For this review, take the finished solid that the model builds, in its own axes (mm). Coordinates: 2 decimals unless noted, no trailing zeros. Loops run counter-clockwise (first coordinate to the right, second up) from the corner with the lowest first, then second, coordinate; pieces in that order, holes last.
1. Take a section at B-B, the plane z = -371. State the section outline as (x, y) points, then the cut area to 3 significant figures.
2. Clearance check with flat-ended pins moving along their axes: P1, Ø12.5, axis at y = 743.5, z = -1133.5, coming from the +X side; P2, Ø23, axis at x = 364, y = 55, coming from the -Z side; P3, Ø12.5, axis at y = 755, z = -111.5, coming from the -X side. State where each tip first meets the part, or that it passes through.
3. To check wall thickness, follow probe 1 along Y at (x, z) = (1123, -1114); probe 2 along Y at (x, z) = (302, -77); probe 3 along Z at (x, y) = (80, 551). State the ranges of each line that lie inside material, in increasing order.
4. Take a section at C-C, the plane y = 277.5. State the section outline as (x, z) points, then the cut area to 3 significant figures.
5. Take a section at A-A, the plane x = 207.5. State the section outline as (y, z) points.
```python
from build123d import *

# Parameters (mm, degrees)
SKETCH1_W               = 1219.2
SKETCH1_H               = 1219.2
BOSS_EXTRUDE1_DEPTH     = 25.4
SKETCH2_W               = 76.2
SKETCH2_H               = 76.2
BOSS_EXTRUDE2_DEPTH     = 711.2
BOSS_EXTRUDE3_REACH     = 1812.541
SKETCH3_W               = 76.2
SKETCH3_H               = 76.2
BOSS_EXTRUDE4_REACH     = 1812.541
SKETCH4_W               = 76.2
SKETCH4_H               = 76.2
SKETCH5_W               = 127
SKETCH5_H               = 127
BOSS_EXTRUDE5_DEPTH     = 25.4
F_1_2_13_TAPPED_HOLE1_D = 10.71626


with BuildPart() as part:
    # Sketch1 → Boss-Extrude1 (new body)
    with BuildSketch(Plane(origin=(0, 0, 0), x_dir=(1, 0, 0), z_dir=(0, 1, 0))):
        with Locations((609.6, 609.6)):
            Rectangle(SKETCH1_W, SKETCH1_H)
    extrude(amount=BOSS_EXTRUDE1_DEPTH)

    # Sketch2 → Boss-Extrude2 (add)
    with BuildSketch(Plane(origin=(0, 25.4, 0), x_dir=(1, 0, 0), z_dir=(0, 1, 0))):
        with Locations((63.5, 1155.7)):
            Rectangle(SKETCH2_W, SKETCH2_H)
        with Locations((1155.7, 1155.7)):
            Rectangle(SKETCH2_W, SKETCH2_H)
        with Locations((1155.7, 63.5)):
            Rectangle(SKETCH2_W, SKETCH2_H)
        with Locations((63.5, 63.5)):
            Rectangle(SKETCH2_W, SKETCH2_H)
    extrude(amount=BOSS_EXTRUDE2_DEPTH)

    # Sketch3 → Boss-Extrude3 (add, up to next)
    with BuildSketch(Plane(origin=(0, 0, -101.6), x_dir=(-1, 0, 0), z_dir=(0, 0, -1)), mode=Mode.PRIVATE) as boss_extrude3_sk1:
        with Locations((-63.5, 63.5)):
            Rectangle(SKETCH3_W, SKETCH3_H)
    boss_extrude3_tool1 = extrude(boss_extrude3_sk1.sketch, amount=BOSS_EXTRUDE3_REACH, mode=Mode.PRIVATE) - part.part
    # Sketch3 → Boss-Extrude3 (add, up to next)
    with BuildSketch(Plane(origin=(0, 0, -101.6), x_dir=(-1, 0, 0), z_dir=(0, 0, -1)), mode=Mode.PRIVATE) as boss_extrude3_sk2:
        with Locations((-1155.7, 63.5)):
            Rectangle(SKETCH3_W, SKETCH3_H)
    boss_extrude3_tool2 = extrude(boss_extrude3_sk2.sketch, amount=BOSS_EXTRUDE3_REACH, mode=Mode.PRIVATE) - part.part
    # Sketch3 → Boss-Extrude3 (add, up to next)
    with BuildSketch(Plane(origin=(0, 0, -101.6), x_dir=(-1, 0, 0), z_dir=(0, 0, -1)), mode=Mode.PRIVATE) as boss_extrude3_sk3:
        with Locations((-63.5, 622.3)):
            Rectangle(SKETCH3_W, SKETCH3_H)
    boss_extrude3_tool3 = extrude(boss_extrude3_sk3.sketch, amount=BOSS_EXTRUDE3_REACH, mode=Mode.PRIVATE) - part.part
    # Sketch3 → Boss-Extrude3 (add, up to next)
    with BuildSketch(Plane(origin=(0, 0, -101.6), x_dir=(-1, 0, 0), z_dir=(0, 0, -1)), mode=Mode.PRIVATE) as boss_extrude3_sk4:
        with Locations((-1155.7, 622.3)):
            Rectangle(SKETCH3_W, SKETCH3_H)
    boss_extrude3_tool4 = extrude(boss_extrude3_sk4.sketch, amount=BOSS_EXTRUDE3_REACH, mode=Mode.PRIVATE) - part.part
    add(boss_extrude3_tool1.solids().sort_by_distance((63.5, 63.5, -101.6))[0])
    add(boss_extrude3_tool2.solids().sort_by_distance((1155.7, 63.5, -101.6))[0])
    add(boss_extrude3_tool3.solids().sort_by_distance((63.5, 622.3, -101.6))[0])
    add(boss_extrude3_tool4.solids().sort_by_distance((1155.7, 622.3, -101.6))[0])

    # Sketch4 → Boss-Extrude4 (add, up to next)
    with BuildSketch(Plane.ZY.offset(-1117.6), mode=Mode.PRIVATE) as boss_extrude4_sk1:
        with Locations((-63.5, 63.5)):
            Rectangle(SKETCH4_W, SKETCH4_H)
    boss_extrude4_tool1 = extrude(boss_extrude4_sk1.sketch, amount=BOSS_EXTRUDE4_REACH, mode=Mode.PRIVATE) - part.part
    # Sketch4 → Boss-Extrude4 (add, up to next)
    with BuildSketch(Plane.ZY.offset(-1117.6), mode=Mode.PRIVATE) as boss_extrude4_sk2:
        with Locations((-1155.7, 63.5)):
            Rectangle(SKETCH4_W, SKETCH4_H)
    boss_extrude4_tool2 = extrude(boss_extrude4_sk2.sketch, amount=BOSS_EXTRUDE4_REACH, mode=Mode.PRIVATE) - part.part
    # Sketch4 → Boss-Extrude4 (add, up to next)
    with BuildSketch(Plane.ZY.offset(-1117.6), mode=Mode.PRIVATE) as boss_extrude4_sk3:
        with Locations((-63.5, 622.3)):
            Rectangle(SKETCH4_W, SKETCH4_H)
    boss_extrude4_tool3 = extrude(boss_extrude4_sk3.sketch, amount=BOSS_EXTRUDE4_REACH, mode=Mode.PRIVATE) - part.part
    # Sketch4 → Boss-Extrude4 (add, up to next)
    with BuildSketch(Plane.ZY.offset(-1117.6), mode=Mode.PRIVATE) as boss_extrude4_sk4:
        with Locations((-1155.7, 622.3)):
            Rectangle(SKETCH4_W, SKETCH4_H)
    boss_extrude4_tool4 = extrude(boss_extrude4_sk4.sketch, amount=BOSS_EXTRUDE4_REACH, mode=Mode.PRIVATE) - part.part
    add(boss_extrude4_tool1.solids().sort_by_distance((1117.6, 63.5, -63.5))[0])
    add(boss_extrude4_tool2.solids().sort_by_distance((1117.6, 63.5, -1155.7))[0])
    add(boss_extrude4_tool3.solids().sort_by_distance((1117.6, 622.3, -63.5))[0])
    add(boss_extrude4_tool4.solids().sort_by_distance((1117.6, 622.3, -1155.7))[0])

    # Sketch5 → Boss-Extrude5 (add)
    with BuildSketch(Plane(origin=(0, 736.6, 0), x_dir=(1, 0, 0), z_dir=(0, 1, 0))):
        with Locations((82.55, 82.55)):
            Rectangle(SKETCH5_W, SKETCH5_H)
        with Locations((1136.65, 82.55)):
            Rectangle(SKETCH5_W, SKETCH5_H)
        with Locations((1136.65, 1136.65)):
            Rectangle(SKETCH5_W, SKETCH5_H)
        with Locations((82.55, 1136.65)):
            Rectangle(SKETCH5_W, SKETCH5_H)
    extrude(amount=BOSS_EXTRUDE5_DEPTH)

    # 1/2-13 Tapped Hole1 (through all)
    with Locations(Plane(origin=(0, 0, 0), x_dir=(-1, 0, 0), z_dir=(0, -1, 0))):
        with Locations((-673.1, 546.1), (-546.1, 546.1), (-419.1, 546.1), (-292.1, 546.1), (-165.1, 546.1), (-546.1, 419.1), (-419.1, 419.1), (-292.1, 419.1), (-165.1, 419.1), (-546.1, 292.1), (-419.1, 292.1), (-292.1, 292.1), (-165.1, 292.1), (-546.1, 165.1), (-419.1, 165.1), (-292.1, 165.1), (-165.1, 165.1), (-673.1, 419.1), (-673.1, 292.1), (-673.1, 165.1), (-165.1, 673.1), (-673.1, 1054.1), (-673.1, 927.1), (-673.1, 800.1), (-165.1, 1054.1), (-292.1, 1054.1), (-419.1, 1054.1), (-546.1, 1054.1), (-165.1, 927.1), (-292.1, 927.1), (-419.1, 927.1), (-546.1, 927.1), (-165.1, 800.1), (-292.1, 800.1), (-419.1, 800.1), (-546.1, 800.1), (-292.1, 673.1), (-419.1, 673.1), (-546.1, 673.1), (-673.1, 673.1), (-800.1, 673.1), (-927.1, 673.1), (-800.1, 800.1), (-927.1, 800.1), (-1054.1, 800.1), (-800.1, 927.1), (-927.1, 927.1), (-1054.1, 927.1), (-800.1, 1054.1), (-927.1, 1054.1), (-1054.1, 1054.1), (-1054.1, 673.1), (-1054.1, 165.1), (-927.1, 165.1), (-800.1, 165.1), (-1054.1, 292.1), (-927.1, 292.1), (-800.1, 292.1), (-1054.1, 419.1), (-927.1, 419.1), (-800.1, 419.1), (-1054.1, 546.1), (-927.1, 546.1), (-800.1, 546.1)):
            Hole(F_1_2_13_TAPPED_HOLE1_D / 2)


solid = part.part
```
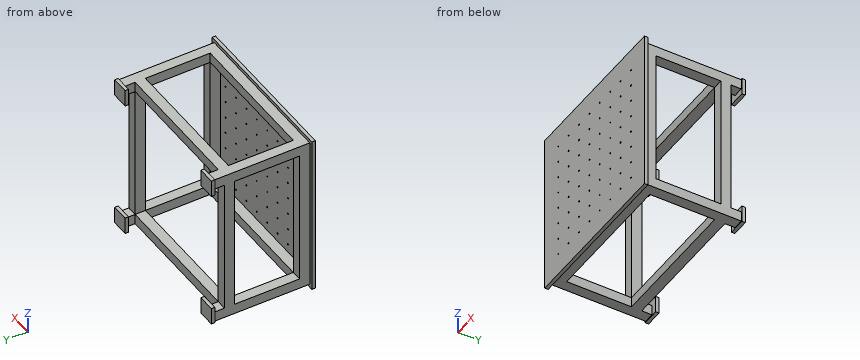
Results list:
1. outline: (0, 0) - (1219.2, 0) - (1219.2, 25.4) - (1193.8, 25.4) - (1193.8, 101.6) - (1117.6, 101.6) - (1117.6, 25.4) - (101.6, 25.4) - (101.6, 101.6) - (25.4, 101.6) - (25.4, 25.4) - (0, 25.4) - close; (25.4, 584.2) - (101.6, 584.2) - (101.6, 660.4) - (25.4, 660.4) - close; (1117.6, 584.2) - (1193.8, 584.2) - (1193.8, 660.4) - (1117.6, 660.4) - close
1. area: 54,200 mm2
2. P1: stops at x = 1200.15
2. P2: stops at z = -1193.8
2. P3: stops at x = 19.05
3. probe 1: y = 0 to 101.6, 584.2 to 660.4, 736.6 to 762
3. probe 2: y = 0 to 101.6, 584.2 to 660.4
3. probe 3: z = -1193.8 to -1117.6, -101.6 to -25.4
4. outline: (25.4, -1193.8) - (101.6, -1193.8) - (101.6, -1117.6) - (25.4, -1117.6) - close; (25.4, -101.6) - (101.6, -101.6) - (101.6, -25.4) - (25.4, -25.4) - close; (1117.6, -1193.8) - (1193.8, -1193.8) - (1193.8, -1117.6) - (1117.6, -1117.6) - close; (1117.6, -101.6) - (1193.8, -101.6) - (1193.8, -25.4) - (1117.6, -25.4) - close
4. area: 23,200 mm2
5. outline: (0, -1219.2) - (25.4, -1219.2) - (25.4, -1193.8) - (101.6, -1193.8) - (101.6, -1117.6) - (25.4, -1117.6) - (25.4, -101.6) - (101.6, -101.6) - (101.6, -25.4) - (25.4, -25.4) - (25.4, 0) - (0, 0) - close; (584.2, -1193.8) - (660.4, -1193.8) - (660.4, -1117.6) - (584.2, -1117.6) - close; (584.2, -101.6) - (660.4, -101.6) - (660.4, -25.4) - (584.2, -25.4) - close
